Here's how the part is built. I have some questions about the finished solid (model axes, mm). Give positions to 0.01 mm unless a question says otherwise; leave off trailing zeros. Loops run counter-clockwise (first coordinate to the right, second up) from the corner with the lowest first, then second, coordinate; pieces in that order, holes last. Notation, with made-up numbers: (-29.75, 42) -> (24.25, 42) arc R25 cw to (24.25, 72) -> close; hole circle Ø7 at (34.5, -14.5). An arc over 180 degrees is marked (long way). Answer in a Markdown table with one row per item. Add a question column.
Item 1: If I drill on line 1 (Y direction, x = 19.05, z = -4); line 2 (X direction, y = 17, z = -2.25); line 3 (X direction, y = 20, z = -0.75), over which ranges is the centre line in solid material (lowest first)?
Item 2: If we section it at A-A (x = 19.05): Write out the boundary of the cut face in (y, z).
Item 3: If we section it at C-C (z = -4.25): Write out the boundary of the cut face in (x, y).
Item 4: We'd pull the mould along X, two halves only. Please class faces 1 (the face through (0, 19, -5)), 2 (the face through (16.24, 21.62, -3.13)), 3 (the face through (19.317, 1.086, -1.146)): released by +X, released by -X, zero draft, split by the parting line, or undercut.
Item 5: If we section it at D-D (x = 31): Write out the boundary of the cut face in (y, z).
```python
from build123d import *

# Parameters (mm, degrees)
F0_W     = 38.1
F0_H     = 38.1
F1_DEPTH = 6.35
F2_R     = 3.81
F3_R     = 3.81
F4_DEPTH = 6.351


with BuildPart() as f1:
    # F0 (on Top) → F1 (new body)
    with BuildSketch(Plane.XY):
        with Locations((19.05, 19.05)):
            Rectangle(F0_W, F0_H)
    extrude(amount=-F1_DEPTH)

    # F2
    f2_edges = [f1.edges().sort_by_distance(p)[0] for p in [
        (0, 19.05, 0),
        (19.05, 0, 0),
        (38.1, 19.05, 0),
        (19.05, 38.1, 0),
    ]]
    fillet(f2_edges, radius=F2_R)

    # F3 (on face) → F4 (cut, through all)
    with BuildSketch(Plane.XY):
        with Locations((19.05, 19.05)):
            Circle(F3_R)
    extrude(amount=-F4_DEPTH, mode=Mode.SUBTRACT)


solid = f1.part
```
Recorded:
| question | item | result |
|---|---|---|
| 1 | line 1 | y = 0 to 15.24, 22.86 to 38.1 |
| 1 | line 2 | x = 0.33 to 15.84, 22.26 to 37.77 |
| 1 | line 3 | x = 1.54 to 15.36, 22.74 to 36.56 |
| 2 | outline | (0, -6.35) -> (15.24, -6.35) -> (15.24, 0) -> (3.81, 0) arc R3.81 ccw to (0, -3.81) -> close; (22.86, -6.35) -> (38.1, -6.35) -> (38.1, -3.81) arc R3.81 ccw to (34.29, 0) -> (22.86, 0) -> close |
| 3 | outline | (0, 0) -> (38.1, 0) -> (38.1, 38.1) -> (0, 38.1) -> close; hole circle Ø7.62 at (19.05, 19.05) |
| 4 | face 1 | released by -X |
| 4 | face 2 | undercut |
| 4 | face 3 | zero draft |
| 5 | outline | (0, -6.35) -> (38.1, -6.35) -> (38.1, -3.81) arc R3.81 ccw to (34.29, 0) -> (3.81, 0) arc R3.81 ccw to (0, -3.81) -> close |
